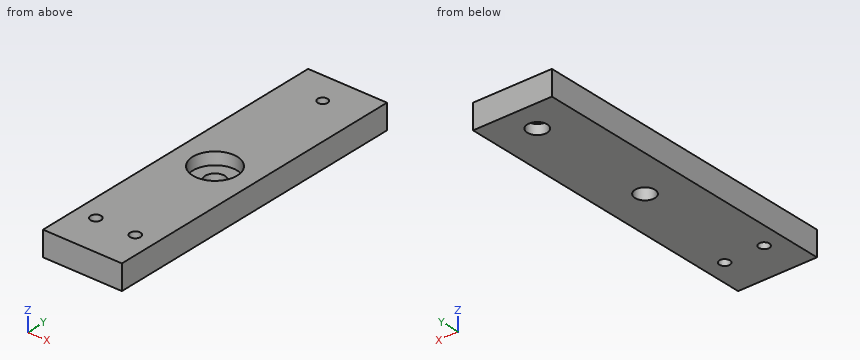
from build123d import *

# Parameters (mm, degrees)
SKETCH1_W                   = 50.8
SKETCH1_H                   = 203.2
BOSS_EXTRUDE1_DEPTH         = 15.875
SKETCH2_R                   = 3.3782
CUT_EXTRUDE1_DEPTH          = 16.875
SKETCH5_R                   = 6.35
CUT_EXTRUDE2_DEPTH          = 6.35
F_1_4_0_25_DIAMETER_HOLE1_D = 6.35
SKETCH5_3_R                 = 6.35
CUT_EXTRUDE3_DEPTH          = 16.875
SKETCH10_R                  = 14.2875
SKETCH10_R_2                = 6.35
CUT_EXTRUDE4_DEPTH          = 7.9375


with BuildPart() as part:
    # Sketch1 → Boss-Extrude1 (new body)
    with BuildSketch(Plane.XY):
        with Locations((0, 76.2)):
            Rectangle(SKETCH1_W, SKETCH1_H)
    extrude(amount=BOSS_EXTRUDE1_DEPTH)

    # Sketch2 → Cut-Extrude1 (cut, through all)
    with BuildSketch(Plane.XY.offset(15.875)):
        with Locations((-12.7, 0)):
            Circle(SKETCH2_R)
        with Locations((12.7, 0)):
            Circle(SKETCH2_R)
    extrude(amount=-CUT_EXTRUDE1_DEPTH, mode=Mode.SUBTRACT)

    # Sketch5 → Cut-Extrude2 (cut)
    with BuildSketch(Plane(origin=(0, 0, 0), x_dir=(-1, 0, 0), z_dir=(0, 0, -1))):
        with Locations((0, 158.75)):
            Circle(SKETCH5_R)
    extrude(amount=-CUT_EXTRUDE2_DEPTH, mode=Mode.SUBTRACT)

    # 1_4 _0.25_ Diameter Hole1 (through all)
    with Locations(Plane(origin=(0, 0, 6.35), x_dir=(-1, 0, 0), z_dir=(0, 0, -1))):
        with Locations((0, 158.75)):
            Hole(F_1_4_0_25_DIAMETER_HOLE1_D / 2)

    # Sketch5_3 → Cut-Extrude3 (cut, through all)
    with BuildSketch(Plane(origin=(0, 0, 0), x_dir=(-1, 0, 0), z_dir=(0, 0, -1))):
        with Locations((0, 76.2)):
            Circle(SKETCH5_3_R)
    extrude(amount=-CUT_EXTRUDE3_DEPTH, mode=Mode.SUBTRACT)

    # Sketch10 → Cut-Extrude4 (cut)
    with BuildSketch(Plane.XY.offset(15.875)):
        with Locations((0, 76.2)):
            Circle(SKETCH10_R)
        with Locations((0, 76.2)):
            Circle(SKETCH10_R_2, mode=Mode.SUBTRACT)
    extrude(amount=-CUT_EXTRUDE4_DEPTH, mode=Mode.SUBTRACT)


solid = part.part
Can you work these out from the model? Positions are in its coordinate system, mm. Coordinates: 2 decimals unless noted, no trailing zeros. Loops run counter-clockwise (first coordinate to the right, second up) from the corner with the lowest first, then second, coordinate; pieces in that order, holes last. Notation, with made-up numbers: (35, 56.25) - (84, 56.25) arc R15 ccw to (84, 74.25) - close; hole circle Ø7 at (65, 7.5). An arc over 180 degrees is marked (long way). Put each result on its own line as item: value. Start each with the question number.
Item 1: Suppose I cut it at C-C (z = 2.25). Please give me the cut outline in (x, y), and give its area (4 significant figures).
Item 2: If I drill on line 1 along Y through (x, z) = (0, 13) (1 decimal); line 2 along Y through (x, z) = (0, 3.5); line 3 along X through (y, z) = (76.2, 4.75), over which ranges is the centre line in solid material (lowest first)?
Item 3: Suppose I cut it at A-A (x = 0). State how many separate pieces and enclosed holes the cut face has, and give its area (3 significant figures).
Item 4: For pin 1 (4 mm diameter, centred on x = 0, y = 158.75, fed in from -Z); pin 2 (16.5 mm diameter, centred on x = 0, y = 76.2, fed in from +Z); pin 3 (7.5 mm diameter, centred on x = 0, y = 158.75, fed in from -Z), each with a flat end and sliding along its axis, tell me the tip position at first contact or that it passes through.
Here are the results:
1. outline: (-25.4, -25.4) - (25.4, -25.4) - (25.4, 177.8) - (-25.4, 177.8) - close; hole circle Ø6.76 at (-12.7, 0); hole circle Ø12.7 at (0, 76.2); hole circle Ø12.7 at (0, 158.75); hole circle Ø6.76 at (12.7, 0)
1. area: 10,000 mm²
2. line 1: -25.4 to 61.9, 90.5 to 155.6, 161.9 to 177.8
2. line 2: -25.4 to 69.85, 82.55 to 152.4, 165.1 to 177.8
2. line 3: -25.4 to -6.35, 6.35 to 25.4
3. separate pieces: 3
3. enclosed holes: 0
3. area: 2,760 mm²
4. pin 1: through
4. pin 2: z = 7.94
4. pin 3: z = 6.35
